```python
from build123d import *

# Parameters (mm, degrees)
SKETCH1_W           = 120
SKETCH1_H           = 100
BOSS_EXTRUDE1_DEPTH = 75
SKETCH2_W           = 100
SKETCH2_H           = 100
CUT_EXTRUDE1_DEPTH  = 40
SKETCH6_W           = 15.5
SKETCH6_H           = 15.5
CUT_EXTRUDE4_DEPTH  = 100
SKETCH8_W           = 19.1
SKETCH8_H           = 10
CUT_EXTRUDE5_DEPTH  = 100
SKETCH6_3_R         = 5.95
CUT_EXTRUDE6_DEPTH  = 111
FILLET1_R           = 1
CHAMFER1_SIZE       = 1
FILLET2_R           = 0.5


with BuildPart() as part:
    # Sketch1 → Boss-Extrude1 (new body)
    with BuildSketch(Plane(origin=(0, 0, 0), x_dir=(1, 0, 0), z_dir=(0, 1, 0))):
        with Locations((-3.53539823, -7.581858407)):
            Rectangle(SKETCH1_W, SKETCH1_H)
    extrude(amount=BOSS_EXTRUDE1_DEPTH)

    # Sketch2 → Cut-Extrude1 (cut)
    with BuildSketch(Plane(origin=(0, 75, 0), x_dir=(1, 0, 0), z_dir=(0, 1, 0))):
        with Locations((-13.53539823, -7.581858407)):
            Rectangle(SKETCH2_W, SKETCH2_H)
    extrude(amount=-CUT_EXTRUDE1_DEPTH, mode=Mode.SUBTRACT)

    # Sketch6 → Cut-Extrude4 (cut)
    with BuildSketch(Plane.ZY.offset(63.53539823)):
        with Locations((-27.068141593, 27.25)):
            Rectangle(SKETCH6_W, SKETCH6_H)
        with Locations((-3.968141593, 27.25)):
            Rectangle(SKETCH6_W, SKETCH6_H)
        with Locations((19.131858407, 27.25)):
            Rectangle(SKETCH6_W, SKETCH6_H)
        with Locations((42.231858407, 27.25)):
            Rectangle(SKETCH6_W, SKETCH6_H)
    extrude(amount=-CUT_EXTRUDE4_DEPTH, mode=Mode.SUBTRACT)

    # Sketch8 → Cut-Extrude5 (cut)
    with BuildSketch(Plane.ZY.offset(63.53539823)):
        with Locations((-27.068141593, 14.5)):
            Rectangle(SKETCH8_W, SKETCH8_H)
        with Locations((-3.968141593, 14.5)):
            Rectangle(SKETCH8_W, SKETCH8_H)
        with Locations((42.231858407, 14.5)):
            Rectangle(SKETCH8_W, SKETCH8_H)
        with Locations((19.131858407, 14.5)):
            Rectangle(SKETCH8_W, SKETCH8_H)
    extrude(amount=-CUT_EXTRUDE5_DEPTH, mode=Mode.SUBTRACT)

    # Sketch6<3> → Cut-Extrude6 (cut)
    with BuildSketch(Plane.ZY.offset(63.53539823)):
        with Locations((-27.068141593, 27.25)):
            Circle(SKETCH6_3_R)
        with Locations((-3.968141593, 27.25)):
            Circle(SKETCH6_3_R)
        with Locations((42.231858407, 27.25)):
            Circle(SKETCH6_3_R)
        with Locations((19.131858407, 27.25)):
            Circle(SKETCH6_3_R)
    extrude(amount=-CUT_EXTRUDE6_DEPTH, mode=Mode.SUBTRACT)

    # Fillet1
    fillet1_edges = [part.edges().sort_by_distance(p)[0] for p in [
        (56.46460177, 75, 7.581858407),
        (46.46460177, 75, 57.581858407),
        (46.46460177, 75, -42.418141593),
        (-13.53539823, 35, -42.418141593),
        (36.46460177, 55, -42.418141593),
        (-13.53539823, 35, 57.581858407),
        (36.46460177, 55, 57.581858407),
        (36.46460177, 75, 7.581858407),
        (56.46460177, 37.5, -42.418141593),
        (56.46460177, 37.5, 57.581858407),
    ]]
    fillet(fillet1_edges, radius=FILLET1_R)

    # Chamfer1
    chamfer1_edges = [part.edges().sort_by_distance(p)[0] for p in [
        (36.46460177, 27.25, -33.018141593),
        (36.46460177, 27.25, -9.918141593),
        (36.46460177, 27.25, 13.181858407),
        (36.46460177, 27.25, 36.281858407),
    ]]
    chamfer(chamfer1_edges, length=CHAMFER1_SIZE)

    # Fillet2
    fillet2_edges = [part.edges().sort_by_distance(p)[0] for p in [
        (47.46460177, 27.25, -33.018141593),
        (47.46460177, 27.25, -9.918141593),
        (47.46460177, 27.25, 13.181858407),
        (47.46460177, 27.25, 36.281858407),
    ]]
    fillet(fillet2_edges, radius=FILLET2_R)


solid = part.part
```
Model file for the job. Use its own axes, mm. A direction names the side the tool comes from. Coordinates: 2 decimals unless noted, no trailing zeros. Write each loop counter-clockwise with the first axis right and the second up, starting at its lowest first coordinate (ties: lowest second). Pieces come first, ordered by that corner, then holes. Notation, with made-up numbers: (-27, 89.5) - (31, 89.5) arc R21 ccw to (31, 110.5) - close; hole circle Ø5 at (3, 6.25). An arc over 180 degrees is marked (long way). One line per item, written item: value. Start each with the question number.
1. Probe line 1 (Z direction, x = -0.5, y = 12); line 2 (Y direction, x = 28, z = 4); line 3 (X direction, y = 58, z = 8.5). List the from-to ranges inside material, lowest first. Write a range as from..to.
2. Slice it at A-A (x = 42). Write the cut outline in (y, z), plus the area to 3 significant figures.
3. Tool access for faces 1 (the flat face through (47.465, 27, 42)), 2 (the flat face through (-14, 35, 53)): list every direction of +Z, -Z, +X, -X, +Y, -Y with a clear straight run to the whole face (end or side of a thin tool).
4. Slice it at B-B (y = 61). Write the cut outline in (x, z).
5. Mould opens along Z. For faces 3 (the flat face through (-5, 20, 57.582)), 4 (the flat face through (-14, 14, 51.782)), 5 (the flat face through (-63.535, 13, 8)) say: released by +Z, released by -Z, zero draft, split by the parting line, or undercut.
6. Flat gauge pins, fed straight in: pin 1 (10 mm diameter, centred on x = -15.5, z = 37, fed in from +Y); pin 2 (8.5 mm diameter, centred on y = 27.5, z = 21, fed in from -X); pin 3 (1 mm diameter, centred on x = 2.5, z = 23, fed in from +Y). Where does each tip first touch, or does it go through?
Answers below:
1. line 1: z = -42.42..-36.62, -17.52..-13.52, 5.58..9.58, 28.68..32.68, 51.78..57.58
1. line 2: y = 0..9.5, 19.5..35
1. line 3: x = 36.46..56.46
2. outline: (0, -42.42) - (74, -42.42) arc R1 ccw to (75, -41.42) - (75, 56.58) arc R1 ccw to (74, 57.58) - (0, 57.58) - close; hole circle Ø11.9 at (27.25, -27.07); hole circle Ø11.9 at (27.25, -3.97); hole circle Ø11.9 at (27.25, 19.13); hole circle Ø11.9 at (27.25, 42.23)
2. area: 7,050 mm^2
3. face 1: -X
3. face 2: +Z, -Z, -X, +Y
4. outline: (36.46, -41.42) arc R1 ccw to (37.46, -42.42) - (55.46, -42.42) arc R1 ccw to (56.46, -41.42) - (56.46, 56.58) arc R1 ccw to (55.46, 57.58) - (37.46, 57.58) arc R1 ccw to (36.46, 56.58) - close
5. face 3: released by +Z
5. face 4: undercut
5. face 5: zero draft
6. pin 1: stops at y = 35
6. pin 2: stops at x = 37.28
6. pin 3: stops at y = 9.5
